from build123d import *

# Parameters (mm, degrees)
F1_DEPTH = 9.525


with BuildPart() as f1:
    # F0 (on Top) → F1 (new body, symmetric)
    with BuildSketch(Plane.XY):
        with BuildLine():
            Line((1164.285257, 41.734285), (97.485257, 41.734285))
            Line((97.485257, 41.734285), (97.485257, -53.515715))
            Line((97.485257, -53.515715), (326.085257, -53.515715))
            Line((326.085257, -53.515715), (326.085257, -142.415715))
            Line((326.085257, -142.415715), (199.085257, -142.415715))
            Line((199.085257, -142.415715), (199.085257, -161.465715))
            Line((199.085257, -161.465715), (97.485257, -161.465715))
            Line((97.485257, -161.465715), (97.485257, -256.715715))
            Line((97.485257, -256.715715), (1164.285257, -256.715715))
            ThreePointArc((1164.285257, -256.715715), (1270.91989, -213.195534), (1316.65218, -107.490715))
            ThreePointArc((1316.65218, -107.490715), (1270.91989, -1.785896), (1164.285257, 41.734285))
        make_face()
    extrude(amount=F1_DEPTH, both=True)


solid = f1.part
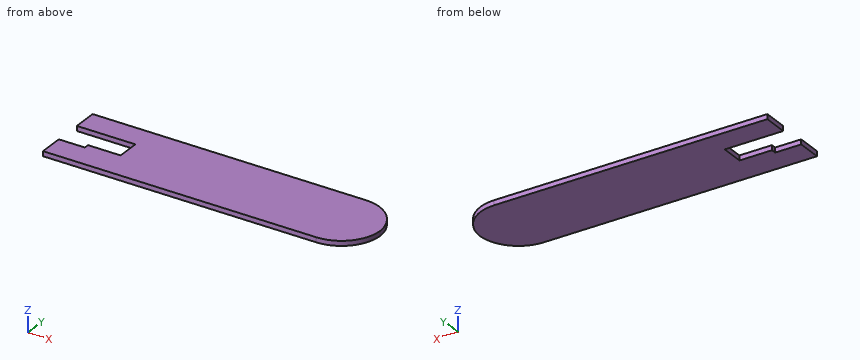
Design review of the part built by this model. Coordinates are the model's own, in mm. Round coordinates to 2 decimals unless told otherwise and drop trailing zeros. Order: outer loops, then holes, each group sorted by start corner. A loop starts at its lowest first (then second) coordinate and runs counter-clockwise, first axis right, second up.
1) Consider section D-D (x = 1212.5). State the section outline as (y, z) points (3 decimals).
The answers:
outline: (-248.888, -9.525) - (33.906, -9.525) - (33.906, 9.525) - (-248.888, 9.525) - close
2) For L1, parallel to Y at x = 253, z = -7.25; L2, parallel to Y at x = 170, z = 2.75; L3, parallel to X at y = -234, z = -8.25, list the stretches that pass through material, from the lowest coordinate up.
The answers:
L1: y = -256.72 to -142.42, -53.52 to 41.73
L2: y = -256.72 to -161.47, -53.52 to 41.73
L3: x = 97.49 to 1244.33
3) Consider section A-A (x = 216). State the section outline as (y, z) points (3 decimals), plus the area to 3 significant figures.
The answers:
outline: (-256.716, -9.525) - (-142.416, -9.525) - (-142.416, 9.525) - (-256.716, 9.525) - close; (-53.516, -9.525) - (41.734, -9.525) - (41.734, 9.525) - (-53.516, 9.525) - close
area: 3,990 mm2
4) Consider section C-C (y = -11.5). State the section outline as (x, z) points (3 decimals), plus the area to 3 significant figures.
The answers:
outline: (97.485, -9.525) - (1280.009, -9.525) - (1280.009, 9.525) - (97.485, 9.525) - close
area: 22,500 mm2
5) Clearance check with flat-ended pins moving along their axes: pin 1 Ø8 at (y, z) = (-149.5, -6.5) entering from -X; pin 2 Ø5.5 at (y, z) = (-87, 0) entering from -X. State where each tip first meets the part, or that it passes through.
The answers:
pin 1: stops at x = 199.09
pin 2: stops at x = 326.09
6) Consider section B-B (z = -5.25). State the section outline as (x, y) points.
The answers:
outline: (97.49, -256.72) - (1164.29, -256.72) arc R152.4 ccw to (1316.65, -107.49) arc R152.4 ccw to (1164.29, 41.73) - (97.49, 41.73) - (97.49, -53.52) - (326.09, -53.52) - (326.09, -142.42) - (199.09, -142.42) - (199.09, -161.47) - (97.49, -161.47) - close
